from build123d import *

# Parameters (mm, degrees)
ESQUISSE1_R             = 2.6
BOSS_EXTRU_1_DEPTH      = 8
ESQUISSE3_R             = 5.1
ENL_V_MAT_EXTRU_2_DEPTH = 4
ESQUISSE4_R             = 5.5
ESQUISSE4_R_2           = 4.5
ENL_V_MAT_EXTRU_3_DEPTH = 2
CONG_1_R                = 5
CONG_2_R                = 3
CONG_3_R                = 4


with BuildPart() as part:
    # Esquisse1 → Boss.-Extru.1 (new body)
    with BuildSketch(Plane(origin=(0, 0, 0), x_dir=(1, 0, 0), z_dir=(0, 1, 0))):
        Polygon((-35, 0), (35, 0), (35, 6), (20, 21), (15, 21), (15, 5), (-15, 5), (-15, 21), (-20, 21), (-35, 6), align=None)
        with Locations((22.5, 7.5)):
            Circle(ESQUISSE1_R, mode=Mode.SUBTRACT)
        with Locations((-22.5, 7.5)):
            Circle(ESQUISSE1_R, mode=Mode.SUBTRACT)
    extrude(amount=BOSS_EXTRU_1_DEPTH)

    # Esquisse3 → Enlèv. mat.-Extru.2 (cut)
    with BuildSketch(Plane(origin=(0, 8, 0), x_dir=(1, 0, 0), z_dir=(0, 1, 0))):
        with Locations((-22.5, 7.5)):
            Circle(ESQUISSE3_R)
        with Locations((22.5, 7.5)):
            Circle(ESQUISSE3_R)
    extrude(amount=-ENL_V_MAT_EXTRU_2_DEPTH, mode=Mode.SUBTRACT)

    # Esquisse4 → Enlèv. mat.-Extru.3 (cut)
    with BuildSketch(Plane.XZ):
        with Locations((-22.5, -7.5)):
            Circle(ESQUISSE4_R)
        with Locations((-22.5, -7.5)):
            Circle(ESQUISSE4_R_2, mode=Mode.SUBTRACT)
        with Locations((22.5, -7.5)):
            Circle(ESQUISSE4_R)
        with Locations((22.5, -7.5)):
            Circle(ESQUISSE4_R_2, mode=Mode.SUBTRACT)
    extrude(amount=-ENL_V_MAT_EXTRU_3_DEPTH, mode=Mode.SUBTRACT)

    # Congé1
    cong_1_edges = [part.edges().sort_by_distance(p)[0] for p in [
        (-35, 4, -6),
        (-20, 4, -21),
        (20, 4, -21),
        (35, 4, -6),
    ]]
    fillet(cong_1_edges, radius=CONG_1_R)

    # Congé2
    cong_2_edges = [part.edges().sort_by_distance(p)[0] for p in [
        (-15, 4, -21),
        (15, 4, -21),
    ]]
    fillet(cong_2_edges, radius=CONG_2_R)

    # Congé3
    cong_3_edges = [part.edges().sort_by_distance(p)[0] for p in [
        (-35, 4, 0),
        (35, 4, 0),
    ]]
    fillet(cong_3_edges, radius=CONG_3_R)


solid = part.part
Source: CAD feature listing. Evaluate the final solid. Frame: model axes, mm. A direction names the side the tool comes from. Coordinates: 2 decimals unless noted, no trailing zeros. Loops run counter-clockwise (first coordinate to the right, second up) from the corner with the lowest first, then second, coordinate; pieces in that order, holes last. Notation, with made-up numbers: (83, 57) - (124, 57) arc R19 cw to (124, 78) - close; hole circle Ø11 at (-34, -17). An arc over 180 degrees is marked (long way). One line per question, with ' | ' between items.
1) Set-up query: faces 5 (the face through (18.7, 6, -10.9)), 6 (the face through (15, 4, -12)), 7 (the face through (25, 1, -12.4)). Return all of +Z, -Z, +X, -X, +Y, -Y with unobstructed straight access to the full face (end or side cutting, diameter ignored); none if empty.
Report:
face 5: +Y | face 6: -Z, +Y, -Y | face 7: -Y
2) Section C-C, the plane y = 1. Give the number of separate pieces and of enclosed holes in the cut face, then the cut area to 3 significant figures.
Report:
separate pieces: 3 | enclosed holes: 4 | area: 647 mm²
3) Section B-B, the plane x = -22.5. Return loops of the section in (y, z).
Report:
outline: (0, -18.5) - (8, -18.5) - (8, -12.6) - (4, -12.6) - (4, -10.1) - (0, -10.1) - (0, -12) - (2, -12) - (2, -13) - (0, -13) - close; (0, -4.9) - (4, -4.9) - (4, -2.4) - (8, -2.4) - (8, 0) - (0, 0) - (0, -2) - (2, -2) - (2, -3) - (0, -3) - close
4) Section A-A, the plane z = -15.75. Return loops of the section in (x, y).
Report:
outline: (-25.25, 0) - (-15, 0) - (-15, 8) - (-25.25, 8) - close; (15, 0) - (25.25, 0) - (25.25, 8) - (15, 8) - close
5) Line query: line 1 along Z through (x, y) = (-22.5, 0.85); line 2 along X through (y, z) = (5.5, -10.5); line 3 along X through (y, z) = (7.05, -7.5). Output: solid intervals per line, ascending.
Report:
line 1: z = -18.5 to -13, -12 to -10.1, -4.9 to -3, -2 to 0 | line 2: x = -30.5 to -26.62, -18.38 to -15, 15 to 18.38, 26.62 to 30.5 | line 3: x = -33.5 to -27.6, -17.4 to -15, 15 to 17.4, 27.6 to 33.5
6) Pull-direction query (Z, two-part tool) for faces 1 (the face through (-27, 4, -14)), 2 (the face through (0, 4, 0)), 3 (the face through (-26.3, 6, -10.9)), 4 (the face through (-15, 4, -11)); classes: released by +Z, released by -Z, zero draft, split by the parting line, or undercut.
Report:
face 1: released by -Z | face 2: released by +Z | face 3: undercut | face 4: zero draft
7) First-contact query: P1, Ø2, axis at y = 5, z = -9, coming from the +X side; P2, Ø8, axis at x = 22.5, z = -7.5, coming from the +Y side; P3, Ø4, axis at x = 3, y = 3, coming from the -Z side. Flat tips, straight axial feed; report the tip coordinate or a pass-through.
Report:
P1: stops at x = 33 | P2: stops at y = 4 | P3: stops at z = -5
